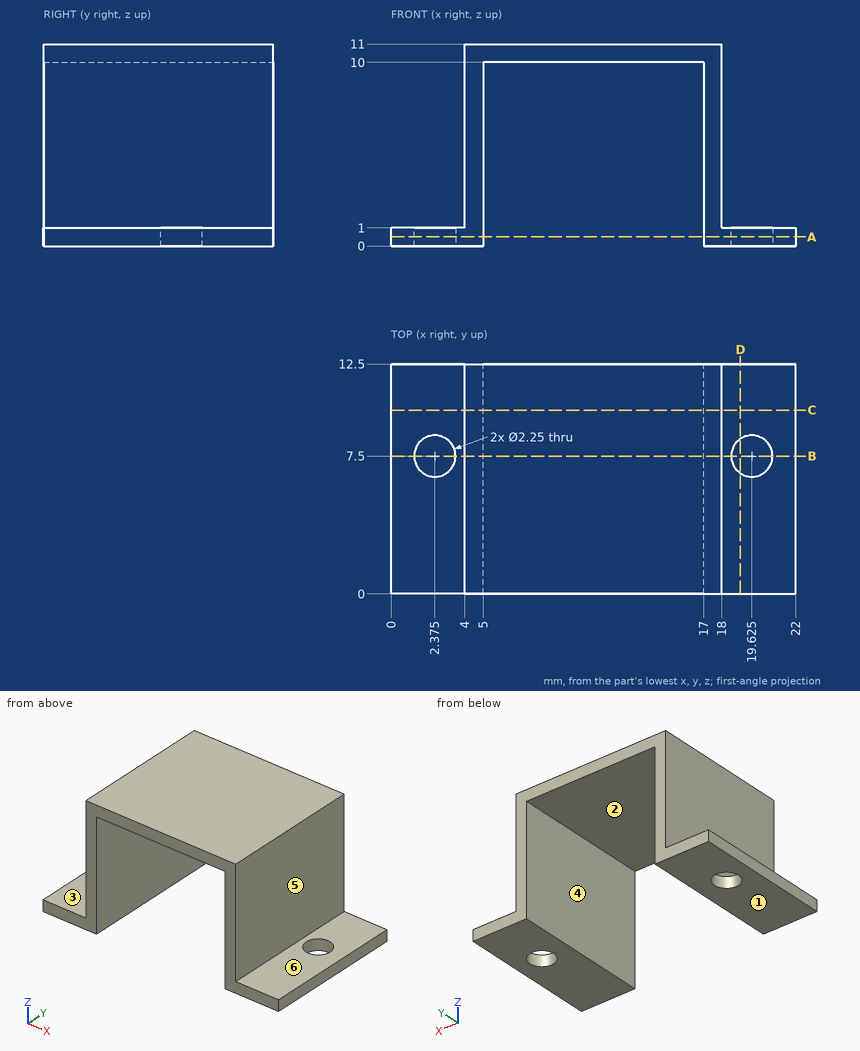
Study the drawing (mm; zero at the part's minimum x, y, z) and answer. A direction names the side the tool comes from. Coordinates: 2 decimals unless noted, no trailing zeros. Loops run counter-clockwise (first coordinate to the right, second up) from the corner with the lowest first, then second, coordinate; pieces in that order, holes last. Notation, with made-up numbers: (29.5, -17) -> (34.5, -17) arc R16 ccw to (34.5, -6) -> close; hole circle Ø3 at (14, 31.25). An arc over 180 degrees is marked (long way). Write each question's results on one line, items separated by ' | '. Start each with the question number.
1) Find section B-B on y = 7.5. Determine the outline of the cut face in (x, z).
2) Consider line 1 along X through (y, z) = (4.75, 2.5); line 2 along X through (y, z) = (2, 0.5); line 3 along Z through (x, y) = (6, 9). Determine where each line is inside the solid, lowest interval first.
3) Find section D-D on x = 19. Determine the outline of the cut face in (y, z), then the cut area to 3 significant figures.
4) Find section A-A on z = 0.5. Determine the outline of the cut face in (x, y) (3 decimals).
5) Find section C-C on y = 10. Determine the outline of the cut face in (x, z), then the cut area to 3 significant figures.
6) Flat-ended cylindrical pins translate along their axes: P1, Ø3, axis at y = 4.5, z = 5, coming from the -X side; P2, Ø1.2, axis at x = 20.5, y = 6, coming from the +Z side; P3, Ø3, axis at y = 5, z = 5.5, coming from the +X side; P4, Ø4, axis at x = 16, z = 5.5, coming from the -Y side. Find the tip coordinate at first contact, or state that the pin passes through.
7) For the marked faces 1, 2 and 3, determine the directions among +Z, -Z, +X, -X, +Y, -Y from which every point of the face is accessible in a straight line to the end or side of a thin tool.
8) The mould has two halves that part along X. Classify the marked faces 4, 5 and 6: pulls with the +X half, pulls with the -X half, needs draft (parallel to the pull), parting line crosses it, or undercut.
Response values:
1) outline: (0, 0) -> (1.25, 0) -> (1.25, 1) -> (0, 1) -> close; (3.5, 0) -> (5, 0) -> (5, 10) -> (17, 10) -> (17, 0) -> (18.5, 0) -> (18.5, 1) -> (18, 1) -> (18, 11) -> (4, 11) -> (4, 1) -> (3.5, 1) -> close; (20.75, 0) -> (22, 0) -> (22, 1) -> (20.75, 1) -> close
2) line 1: x = 4 to 5, 17 to 18 | line 2: x = 0 to 5, 17 to 22 | line 3: z = 10 to 11
3) outline: (0, 0) -> (6.56, 0) -> (6.56, 1) -> (0, 1) -> close; (8.44, 0) -> (12.5, 0) -> (12.5, 1) -> (8.44, 1) -> close | area: 10.6 mm^2
4) outline: (0, 0) -> (5, 0) -> (5, 12.5) -> (0, 12.5) -> close; (17, 0) -> (22, 0) -> (22, 12.5) -> (17, 12.5) -> close; hole circle Ø2.25 at (2.375, 7.5); hole circle Ø2.25 at (19.625, 7.5)
5) outline: (0, 0) -> (5, 0) -> (5, 10) -> (17, 10) -> (17, 0) -> (22, 0) -> (22, 1) -> (18, 1) -> (18, 11) -> (4, 11) -> (4, 1) -> (0, 1) -> close | area: 42.0 mm^2
6) P1: stops at x = 4 | P2: stops at z = 1 | P3: stops at x = 18 | P4: stops at y = 0
7) face 1: -Z, +X, -X, +Y, -Y | face 2: -Z, +Y, -Y | face 3: +Z, -X, +Y, -Y
8) face 4: undercut | face 5: pulls with the +X half | face 6: needs draft
